```python
from build123d import *

# Parameters (mm, degrees)
SKETCH1_W                                       = 200
SKETCH1_H                                       = 170
F_1_4_STEEL_PLATE_DEPTH                         = 6.35
SKETCH2_W                                       = 19.812
SKETCH2_H                                       = 6.604
BLADEHINGECUT_DEPTH                             = 0.635
BLADEHINGEHOLE_D                                = 3.556
SKETCH5_W                                       = 5.05
SKETCH5_H                                       = 5.05
BLADENUTCUT_DEPTH                               = 2
SKETCH6_W                                       = 28
SKETCH6_H                                       = 40
CUT_EXTRUDE1_DEPTH                              = 6.35
SKETCH7_W                                       = 30
SKETCH7_H                                       = 10
SKETCH7_W_2                                     = 10
SKETCH7_H_2                                     = 40
SKETCH7_H_3                                     = 30
SKETCH7_W_3                                     = 40
CUT_EXTRUDE2_DEPTH                              = 5
CUT_EXTRUDE3_START                              = -6.35
SKETCH8_W                                       = 15
SKETCH8_H                                       = 10
CUT_EXTRUDE3_DEPTH                              = 4
CUT_EXTRUDE4_DEPTH                              = 2.35
SKETCH10_W                                      = 15
SKETCH10_H                                      = 10
CUT_EXTRUDE5_DEPTH                              = 4
CUT_EXTRUDE6_REACH                              = 133.305
CSK_FOR_M3_FLAT_HEAD_MACHINE_SCREW1_D           = 3.4
CSK_FOR_M3_FLAT_HEAD_MACHINE_SCREW1_DEPTH       = 14
CSK_FOR_M3_FLAT_HEAD_MACHINE_SCREW1_CSINK_D     = 6.3
CSK_FOR_M3_FLAT_HEAD_MACHINE_SCREW1_CSINK_ANGLE = 90


with BuildPart() as part:
    # Sketch1 → 1/4" Steel Plate (new body)
    with BuildSketch(Plane(origin=(0, 0, 0), x_dir=(1, 0, 0), z_dir=(0, 1, 0))):
        Rectangle(SKETCH1_W, SKETCH1_H)
    extrude(amount=F_1_4_STEEL_PLATE_DEPTH)

    # Sketch2 → BladeHingeCut (cut)
    with BuildSketch(Plane(origin=(0, 6.35, 0), x_dir=(1, 0, 0), z_dir=(0, 1, 0))):
        with Locations((-80.188, -81.698)):
            Rectangle(SKETCH2_W, SKETCH2_H)
    bladehingecut = extrude(amount=-BLADEHINGECUT_DEPTH, mode=Mode.SUBTRACT)

    # BladeHingeHole (through all)
    with Locations(Plane(origin=(-74.6, 5.715, 81.698), x_dir=(0, 0, 1), z_dir=(0, 1, 0))):
        with Locations((0, 0), (0, -11.176)):
            bladehingehole = Hole(BLADEHINGEHOLE_D / 2)

    # Sketch5 → BladeNutCut (cut)
    with BuildSketch(Plane.XZ):
        with Locations((-85.776, 81.698)):
            Rectangle(SKETCH5_W, SKETCH5_H)
        with Locations((-74.6, 81.698)):
            Rectangle(SKETCH5_W, SKETCH5_H)
    bladenutcut = extrude(amount=-BLADENUTCUT_DEPTH, mode=Mode.SUBTRACT)

    # BladeHingeMirror: BladeHingeCut, BladeHingeHole, BladeNutCut across plane
    add(bladehingecut.mirror(Plane.ZY), mode=Mode.SUBTRACT)
    add(bladehingehole.mirror(Plane.ZY), mode=Mode.SUBTRACT)
    add(bladenutcut.mirror(Plane.ZY), mode=Mode.SUBTRACT)

    # Sketch6 → Cut-Extrude1 (cut)
    with BuildSketch(Plane(origin=(0, 0, 0), x_dir=(-1, 0, 0), z_dir=(0, -1, 0))):
        with Locations((68.050545531, -5.523276363)):
            Rectangle(SKETCH6_W, SKETCH6_H)
    cut_extrude1 = extrude(amount=-CUT_EXTRUDE1_DEPTH, mode=Mode.SUBTRACT)

    # Sketch7 → Cut-Extrude2 (cut)
    with BuildSketch(Plane(origin=(0, 0, 0), x_dir=(-1, 0, 0), z_dir=(0, -1, 0))):
        with Locations((68.050545531, -35.523276363)):
            Rectangle(SKETCH7_W, SKETCH7_H)
        with Locations((68.050545531, 24.476723637)):
            Rectangle(SKETCH7_W, SKETCH7_H)
        with Locations((27.050545531, -5.523276363)):
            Rectangle(SKETCH7_W_2, SKETCH7_H_2)
        with Locations((0, -25.523276363)):
            Rectangle(SKETCH7_W, SKETCH7_H)
        with Locations((0, -5.523276363)):
            Rectangle(SKETCH7_W, SKETCH7_H)
        with Locations((0, 14.476723637)):
            Rectangle(SKETCH7_W, SKETCH7_H)
        with Locations((44.050545531, -65.523276363)):
            Rectangle(SKETCH7_W_2, SKETCH7_H_3)
        with Locations((0, -65.523276363)):
            Rectangle(SKETCH7_W_3, SKETCH7_H)
        with Locations((44.050545531, 54.476723637)):
            Rectangle(SKETCH7_W_2, SKETCH7_H_3)
        with Locations((0, 54.476723637)):
            Rectangle(SKETCH7_W_3, SKETCH7_H)
    cut_extrude2 = extrude(amount=-CUT_EXTRUDE2_DEPTH, mode=Mode.SUBTRACT)

    # Sketch8 → Cut-Extrude3 (cut)
    with BuildSketch(Plane(origin=(0, 6.35, 0), x_dir=(1, 0, 0), z_dir=(0, 1, 0)).offset(CUT_EXTRUDE3_START)):
        with Locations((-71.045889297, -68.396)):
            Rectangle(SKETCH8_W, SKETCH8_H)
    cut_extrude3 = extrude(amount=CUT_EXTRUDE3_DEPTH, mode=Mode.SUBTRACT)

    # Sketch9 → Cut-Extrude4 (cut)
    with BuildSketch(Plane.XZ.offset(-4)):
        Polygon((-78.545889297, 63.396), (-63.545889297, 63.396), (-63.545889297, 66.396), (-75.545889297, 66.396), (-75.545889297, 71.396), (-78.545889297, 71.396), align=None)
    cut_extrude4 = extrude(amount=-CUT_EXTRUDE4_DEPTH, mode=Mode.SUBTRACT)

    # Sketch10 → Cut-Extrude5 (cut)
    with BuildSketch(Plane(origin=(0, 0, 0), x_dir=(-1, 0, 0), z_dir=(0, -1, 0))):
        with Locations((67.5, 60)):
            Rectangle(SKETCH10_W, SKETCH10_H)
    cut_extrude5 = extrude(amount=-CUT_EXTRUDE5_DEPTH, mode=Mode.SUBTRACT)

    # Sketch11 → Cut-Extrude6 (cut, up to next)
    with BuildSketch(Plane.XZ.offset(-4), mode=Mode.PRIVATE) as cut_extrude6_sk1:
        Polygon((-60, -55), (-75, -55), (-75, -63), (-72, -63), (-72, -58), (-60, -58), align=None)
    cut_extrude6_tool1 = extrude(cut_extrude6_sk1.sketch, amount=-CUT_EXTRUDE6_REACH, mode=Mode.PRIVATE) & part.part
    cut_extrude6 = cut_extrude6_tool1.solids().sort_by_distance((-69, 4, -57.5))[0]
    add(cut_extrude6, mode=Mode.SUBTRACT)

    # Mirror2: Cut-Extrude1, Cut-Extrude2, Cut-Extrude3, Cut-Extrude4, Cut-Extrude5, Cut-Extrude6 across plane
    add(cut_extrude1.mirror(Plane.ZY), mode=Mode.SUBTRACT)
    add(cut_extrude2.mirror(Plane.ZY), mode=Mode.SUBTRACT)
    add(cut_extrude3.mirror(Plane.ZY), mode=Mode.SUBTRACT)
    add(cut_extrude4.mirror(Plane.ZY), mode=Mode.SUBTRACT)
    add(cut_extrude5.mirror(Plane.ZY), mode=Mode.SUBTRACT)
    add(cut_extrude6.mirror(Plane.ZY), mode=Mode.SUBTRACT)

    # CSK for M3 Flat Head Machine Screw1
    with Locations(Plane(origin=(0, 0, 0), x_dir=(-1, 0, 0), z_dir=(0, -1, 0))):
        with Locations((-91.550289297, -78), (-91.550289297, -62), (-80.337059977, 47.6378), (-80.337059977, 67.6378), (-36.575545542, -6.046552726), (-46.575545542, 33.953447274), (36.575545531, -5), (46.575545531, -45), (91.545889297, -62), (91.545889297, -78), (80.337059966, 47.6378), (80.337059966, 67.6378), (-85.690545542, -20.523276363), (-85.690545542, 9.476723637), (-50.235545542, -20.523276363), (-50.235545542, 9.476723637), (50.235545531, -20.523276363), (85.690545531, -20.523276363), (85.690545531, 9.476723637), (50.235545531, 9.476723637)):
            CounterSinkHole(CSK_FOR_M3_FLAT_HEAD_MACHINE_SCREW1_D / 2, CSK_FOR_M3_FLAT_HEAD_MACHINE_SCREW1_CSINK_D / 2, depth=CSK_FOR_M3_FLAT_HEAD_MACHINE_SCREW1_DEPTH, counter_sink_angle=CSK_FOR_M3_FLAT_HEAD_MACHINE_SCREW1_CSINK_ANGLE)


solid = part.part
```
Here's how the part is built. I have some questions about the finished solid (model axes, mm). A direction names the side the tool comes from. Coordinates: 2 decimals unless noted, no trailing zeros. Order: outer loops, then holes, each group sorted by start corner. A loop starts at its lowest first (then second) coordinate and runs counter-clockwise, first axis right, second up.
1) Imagine slicing it at B-B on x = 67.5. List the corners of the cut face in (y, z) for me, and give its area (3 significant figures).
2) Imagine slicing it at A-A on x = -56.5. List the corners of the cut face in (y, z) for me, and give its area (4 significant figures).
3) Which directions (+Z, -Z, +X, -X, +Y, -Y) give clear straight access to the entire face, cutting with the end or side of a thin tool? Please do faces 3 (the face through (82.051, 3, 6)), 4 (the face through (-63.546, 2, 68)).
4) I need wall thicknesses on line 1 (X direction, y = 5.25, z = 10); line 2 (X direction, y = 4.05, z = 78); line 3 (Z direction, x = 55, y = 4.25). Which ranges of each line are inside material? Lowest first, please.
5) Imagine slicing it at C-C on x = 2. List the corners of the cut face in (y, z) for me, and give its area (4 significant figures).
6) Will these pins go through, and if not, where does the flat tip stop? pin 1 (0.5 mm diameter, centred on x = 77, y = 6, fed in from +Z); pin 2 (2 mm diameter, centred on x = -71.5, z = 71.5, fed in from -Y); pin 3 (4.5 mm diameter, centred on x = -36.58, z = 5, fed in from -Y).
7) We'd pull the mould along X, two halves only. Please class faces 1 (the face through (100, 3, 1)), 2 (the face through (71, 3, 63.396)): +X half, -X half, draft (parallel to the pull), parting line (faces both ways), or undercut.
Response values:
1. outline: (0, -85) - (6.35, -85) - (6.35, -58) - (4, -58) - (4, -65) - (0, -65) - close; (0, -55) - (6.35, -55) - (6.35, -14.48) - (0, -14.48) - (0, -19.48) - (5, -19.48) - (5, -29.48) - (0, -29.48) - close; (0, 25.52) - (6.35, 25.52) - (6.35, 63.4) - (0, 63.4) - (0, 40.52) - (5, 40.52) - (5, 30.52) - (0, 30.52) - close; (0, 73.4) - (4, 73.4) - (4, 66.4) - (6.35, 66.4) - (6.35, 85) - (0, 85) - close
1. area: 631 mm2
2. outline: (0, -85) - (6.35, -85) - (6.35, -14.48) - (0, -14.48) - (0, -19.48) - (5, -19.48) - (5, -29.48) - (0, -29.48) - close; (0, 25.52) - (6.35, 25.52) - (6.35, 85) - (0, 85) - (0, 40.52) - (5, 40.52) - (5, 30.52) - (0, 30.52) - close
2. area: 725.5 mm2
3. face 3: +Y, -Y
3. face 4: -Y
4. line 1: x = -100 to -82.05, -54.05 to 54.05, 82.05 to 100
4. line 2: x = -100 to -93.25, -89.85 to -49.05, -39.05 to 39.05, 49.05 to 89.85, 93.25 to 100
4. line 3: z = -85 to -29.48, -19.48 to -14.48, 25.52 to 30.52, 40.52 to 85
5. outline: (0, -85) - (6.35, -85) - (6.35, 85) - (0, 85) - (0, 70.52) - (5, 70.52) - (5, 60.52) - (0, 60.52) - (0, 30.52) - (5, 30.52) - (5, 20.52) - (0, 20.52) - (0, 10.52) - (5, 10.52) - (5, 0.52) - (0, 0.52) - (0, -9.48) - (5, -9.48) - (5, -19.48) - (0, -19.48) - (0, -49.48) - (5, -49.48) - (5, -59.48) - (0, -59.48) - close
5. area: 829.5 mm2
6. pin 1: stops at z = 78.4
6. pin 2: stops at y = 4
6. pin 3: stops at y = 0.9
7. face 1: +X half
7. face 2: undercut
